from build123d import *

# Parameters (mm, degrees)
SKETCH_1_R      = 2.5
EXTRUDE_1_DEPTH = 10


with BuildPart() as part:
    # 草圖1 → 填料-伸長1 (new body)
    with BuildSketch(Plane.XY):
        with BuildLine():
            Line((-13.71628672, 4.928383), (-17.851865082, -6.434025166))
            ThreePointArc((-17.851865082, -6.434025166), (-17.925532299, -6.592005023), (-18.02551326, -6.734792632))
            Line((-18.02551326, -6.734792632), (-25.315505088, -15.422666584))
            Line((-25.315505088, -15.422666584), (-31.797224631, -20.861475062))
            ThreePointArc((-31.797224631, -20.861475062), (-35.446941393, -22.012226336), (-38.841384895, -20.245190894))
            ThreePointArc((-38.841384895, -20.245190894), (-39.99213617, -16.595474132), (-38.225100728, -13.20103063))
            Line((-38.225100728, -13.20103063), (-15.298766951, 6.036447586))
            ThreePointArc((-15.298766951, 6.036447586), (-14.082402905, 6.089555187), (-13.71628672, 4.928383))
        make_face()
        with Locations((-35.011162679, -17.031252846)):
            Circle(SKETCH_1_R, mode=Mode.SUBTRACT)
    extrude(amount=EXTRUDE_1_DEPTH)


solid = part.part
Part model, mm, in its own coordinate system. Coordinates: 2 decimals unless noted, no trailing zeros. Write each loop counter-clockwise with the first axis right and the second up, starting at its lowest first coordinate (ties: lowest second). Pieces come first, ordered by that corner, then holes. Notation, with made-up numbers: (-40, -35.5) - (-26, -35.5) arc R32 cw to (-26, -9.5) - close; hole circle Ø1 at (40.25, 19.5). An arc over 180 degrees is marked (long way). Put each result on its own line as item: value.
1. Band-saw the part on D-D (x = -21.5). Write the cut outline in (y, z), then the cut area to 3 significant figures.
Final values:
outline: (-10.88, 0) - (0.83, 0) - (0.83, 10) - (-10.88, 10) - close
area: 117 mm²
2. Band-saw the part on A-A (x = -36.75). Write the cut outline in (y, z), then the cut area to 3 significant figures.
Final values:
outline: (-21.72, 0) - (-18.83, 0) - (-18.83, 10) - (-21.72, 10) - close; (-15.24, 0) - (-11.96, 0) - (-11.96, 10) - (-15.24, 10) - close
area: 61.6 mm²
3. Flat gauge pins, fed straight in: pin 1 Ø5 at (x, z) = (-31.5, 2) entering from +Y; pin 2 Ø6 at (y, z) = (-9.5, 7) entering from -X; pin 3 Ø1 at (y, z) = (3, 2.5) entering from -X. Where does each tip first touch, or does it go through?
Final values:
pin 1: stops at y = -5.46
pin 2: stops at x = -37.39
pin 3: stops at x = -19.51
4. Two-plate mould, pull along Y, no slides. Class faces 1 (the flat face through (-15.755, -0.673, 4.93)), 2 (the flat face through (-27, -9, 10)), 3 (the flat face through (-26.9, -3.7, 4.9)), 4 (the cylindrical face through (-32.702, -17.989, 4.93)): +Y half, -Y half, draft (parallel to the pull), parting line (faces both ways), or undercut.
Final values:
face 1: -Y half
face 2: draft
face 3: +Y half
face 4: undercut
5. Probe line 1 along Y through (x, z) = (-36.25, 2.25); line 2 along Y through (x, z) = (-35.25, 2); line 3 along Y through (x, z) = (-23, 7.5). List the from-to ranges inside material, lowest first. Write a range as [from, to].
Final values:
line 1: y = [-21.88, -19.2], [-14.86, -11.54]
line 2: y = [-22.03, -19.52], [-14.54, -10.7]
line 3: y = [-12.66, -0.43]
6. Band-saw the part on C-C (y = -15). Write the cut outline in (x, z), then the cut area to 3 significant figures.
Final values:
outline: (-39.58, 0) - (-36.47, 0) - (-36.47, 10) - (-39.58, 10) - close; (-33.55, 0) - (-24.96, 0) - (-24.96, 10) - (-33.55, 10) - close
area: 117 mm²
7. Band-saw the part on B-B (z = 8). Write the cut outline in (x, y).
Final values:
outline: (-38.23, -13.2) arc R5 ccw to (-31.8, -20.86) - (-25.32, -15.42) - (-18.03, -6.73) arc R1 ccw to (-17.85, -6.43) - (-13.72, 4.93) arc R1 ccw to (-15.3, 6.04) - close; hole circle Ø5 at (-35.01, -17.03)
